from build123d import *

# Parameters (mm, degrees)
SKETCH_1_R      = 4
EXTRUDE_1_DEPTH = 10
SKETCH_2_R      = 5
EXTRUDE_3_DEPTH = 2
SKETCH_4_R      = 5
EXTRUDE_4_DEPTH = 2


with BuildPart() as part:
    # 草图1 → 凸台-拉伸1 (new body)
    with BuildSketch(Plane(origin=(0, 0, 0), x_dir=(1, 0, 0), z_dir=(0, 1, 0))):
        with Locations(Location((-0.063005912, 0, 0), (0, 0, 270))):
            Circle(SKETCH_1_R)
        with BuildLine():
            Line((-1.5, 2), (1.5, 2))
            ThreePointArc((1.5, 2), (0, -2.5), (-1.5, 2))
        make_face(mode=Mode.SUBTRACT)
    extrude(amount=EXTRUDE_1_DEPTH)

    # 草图2 → 凸台-拉伸3 (add)
    with BuildSketch(Plane(origin=(0, 0, 0), x_dir=(1, 0, 0), z_dir=(0, 1, 0))):
        with Locations(Location((0, 0, 0), (0, 0, 270))):
            Circle(SKETCH_2_R)
        with BuildLine():
            Line((-1.5, 2), (1.5, 2))
            ThreePointArc((1.5, 2), (0, -2.5), (-1.5, 2))
        make_face(mode=Mode.SUBTRACT)
    extrude(amount=EXTRUDE_3_DEPTH)

    # 草图4 → 凸台-拉伸4 (add)
    with BuildSketch(Plane(origin=(0, 10, 0), x_dir=(1, 0, 0), z_dir=(0, 1, 0))):
        with Locations(Location((0, 0, 0), (0, 0, 270))):
            Circle(SKETCH_4_R)
        with BuildLine():
            Line((-1.5, 2), (1.5, 2))
            ThreePointArc((1.5, 2), (0, -2.5), (-1.5, 2))
        make_face(mode=Mode.SUBTRACT)
    extrude(amount=EXTRUDE_4_DEPTH)


solid = part.part
Here's how the part is built. I have some questions about the finished solid (model axes, mm). A direction names the side the tool comes from. Give positions to 0.01 mm unless a question says otherwise; leave off trailing zeros. Write each loop counter-clockwise with the first axis right and the second up, starting at its lowest first coordinate (ties: lowest second). Pieces come first, ordered by that corner, then holes. Notation, with made-up numbers: (-9.75, 71.5) -> (-2.75, 71.5) arc R24 cw to (-2.75, 89.5) -> close; hole circle Ø2 at (40, 35). An arc over 180 degrees is marked (long way). Use one line per item in the form item = value. Start each with the question number.
1. Imagine slicing it at A-A on z = 0. List the corners of the cut face in (x, y) for me, plus the area to 3 significant figures.
2. If I drill on L1, parallel to X at y = 4.25, z = 0; L2, parallel to Z at x = 0, y = 8; L3, parallel to Y at x = -3.75, z = -2.25, over which ranges is the centre line in solid material (lowest first)?
3. Thinking about a two-plate mould opening in Z: for faces 1 (the face through (0.1, 12, -2.3)), 2 (the face through (-4.88, 10.99, -1.08)), 3 (the face through (0.1, 5.9, 2.5)), which applies, +Z half, -Z half, draft (parallel to the pull), parting line (faces both ways), or undercut?
4. Will these pins go through, and if not, where does the flat tip stop? pin 1 Ø4 at (x, z) = (-0.5, 1) entering from +Y; pin 2 Ø1 at (y, z) = (2, 1.5) entering from +X; pin 3 Ø1.5 at (x, y) = (-2, 9) entering from +Z; pin 4 Ø0.9 at (x, y) = (-0.5, 3.5) entering from +Z.
5. Imagine slicing it at B-B on y = 10.5. List the corners of the cut face in (x, z) for me, plus the area to 3 significant figures.
6. On a 3-axis mill with a long thin cutter (end or side, diameter ignored), from which of +Z, -Z, +X, -X, +Y, -Y can I reach the whole of each face in a straight line? I mean faces 4 (the face through (0.1, 0, -2.3)), 5 (the face through (4, 10, 1)), 6 (the face through (0, 6, -2)). Say none if no direction works.
7. Imagine slicing it at C-C on z = -2.5. List the corners of the cut face in (x, y) for me.
8. Imagine slicing it at D-D on x = -3. List the corners of the cut face in (y, z) for me, plus the area to 3 significant figures.
Entries:
q1.outline = (-5, 0) -> (-2.5, 0) -> (-2.5, 12) -> (-5, 12) -> (-5, 10) -> (-4.06, 10) -> (-4.06, 2) -> (-5, 2) -> close; (2.5, 0) -> (5, 0) -> (5, 2) -> (3.94, 2) -> (3.94, 10) -> (5, 10) -> (5, 12) -> (2.5, 12) -> close
q1.area = 44.0 mm²
q2.L1 = -4.06 to -2.5, 2.5 to 3.94
q2.L2 = -4 to -2, 2.5 to 4
q2.L3 = 0 to 2, 10 to 12
q3.face_1 = draft
q3.face_2 = parting line
q3.face_3 = undercut
q4.pin_1 = 12
q4.pin_2 = 4.9
q4.pin_3 = 3.82
q4.pin_4 = 4
q5.outline = circle Ø10 at (0, 0); hole (-1.5, -2) -> (1.5, -2) arc R2.5 ccw (long way) to start
q5.area = 59.9 mm²
q6.face_4 = +Z, -Z, +X, -X, -Y
q6.face_5 = none
q6.face_6 = +Y, -Y
q7.outline = (-4.33, 0) -> (4.33, 0) -> (4.33, 2) -> (3.06, 2) -> (3.06, 10) -> (4.33, 10) -> (4.33, 12) -> (-4.33, 12) -> (-4.33, 10) -> (-3.19, 10) -> (-3.19, 2) -> (-4.33, 2) -> close
q8.outline = (0, -4) -> (2, -4) -> (2, -2.72) -> (10, -2.72) -> (10, -4) -> (12, -4) -> (12, 4) -> (10, 4) -> (10, 2.72) -> (2, 2.72) -> (2, 4) -> (0, 4) -> close
q8.area = 75.4 mm²
